Work out the finished part from the listing and answer in its coordinate system (mm). Face numbers are marked on the shaded views. A direction names the side the tool comes from. Round coordinates to 2 decimals unless told otherwise and drop trailing zeros. Loops run counter-clockwise (first coordinate to the right, second up) from the corner with the lowest first, then second, coordinate; pieces in that order, holes last. Notation, with made-up numbers: (-12.5, -27) -> (36.5, -27) arc R25 cw to (36.5, -11) -> close; hole circle Ø7 at (57.25, 84.25). An arc over 180 degrees is marked (long way). Use one line per item in the form item = value.
```python
from build123d import *

# Parameters (mm, degrees)
F0_R     = 6.5
F1_DEPTH = 25
F3_DEPTH = 40
F4_R     = 19.99999
F5_R     = 7
F6_DEPTH = 25


# Not quite as in the source:
# - a fillet or chamfer is up to 0.001 mm smaller than in the source, because OpenCascade refuses the exact size


with BuildPart() as f1:
    # F0 (on Front) → F1 (new body)
    with BuildSketch(Plane.XZ):
        with BuildLine():
            Line((0, -28.0120762104), (0, 51.4879237896))
            Line((0, 51.4879237896), (-45, 51.4879237896))
            Line((-45, 51.4879237896), (-55, 40.4879237896))
            Line((-55, 40.4879237896), (-55, 10.4879237896))
            Line((-55, 10.4879237896), (-22, -51.5120762104))
            Line((-22, -51.5120762104), (0, -51.5120762104))
            Line((0, -51.5120762104), (0, -41.0120762104))
            ThreePointArc((0, -41.0120762104), (-6.5, -34.5120762104), (0, -28.0120762104))
        make_face()
        with Locations((-38, 22.4879237896)):
            Circle(F0_R, mode=Mode.SUBTRACT)
        with BuildLine():
            Line((45, 51.4879237896), (0, 51.4879237896))
            Line((0, 51.4879237896), (0, -28.0120762104))
            ThreePointArc((0, -28.0120762104), (6.5, -34.5120762104), (0, -41.0120762104))
            Line((0, -41.0120762104), (0, -51.5120762104))
            Line((0, -51.5120762104), (22, -51.5120762104))
            Line((22, -51.5120762104), (55, 10.4879237896))
            Line((55, 10.4879237896), (55, 40.4879237896))
            Line((55, 40.4879237896), (45, 51.4879237896))
        make_face()
        with Locations((38, 22.4879237896)):
            Circle(F0_R, mode=Mode.SUBTRACT)
    extrude(amount=F1_DEPTH)

    # F2 (on face) → F3 (join)
    with BuildSketch(Plane(origin=(0, 0, 0), x_dir=(-1, 0, 0), z_dir=(0, 1, 0))):
        Polygon((7, 108.4879237896), (0, 108.4879237896), (-7, 108.4879237896), (-7, 47.4879237896), (-45, 47.4879237896), (-45, 39.4879237896), (-7, 39.4879237896), (-7, -14.5120762104), (0, -14.5120762104), (7, -14.5120762104), (7, 39.4879237896), (45, 39.4879237896), (45, 47.4879237896), (7, 47.4879237896), align=None)
    extrude(amount=F3_DEPTH)

    # F4 (radius 20 in the source; OpenCascade refuses exactly that, so slightly less here)
    f4_edges = [f1.edges().sort_by_distance(p)[0] for p in [
        (0, 0, 108.487924),
        (0, 40, 108.487924),
    ]]
    fillet(f4_edges, radius=F4_R)

    # F5 (on face) → F6 (cut)
    with BuildSketch(Plane.YZ.offset(7)):
        with Locations((20, 88.4879237896)):
            Circle(F5_R)
        Polygon((40, -14.5120762104), (40, 24.4879237896), (17, -14.5120762104), align=None)
    extrude(amount=-F6_DEPTH, mode=Mode.SUBTRACT)


solid = f1.part
```
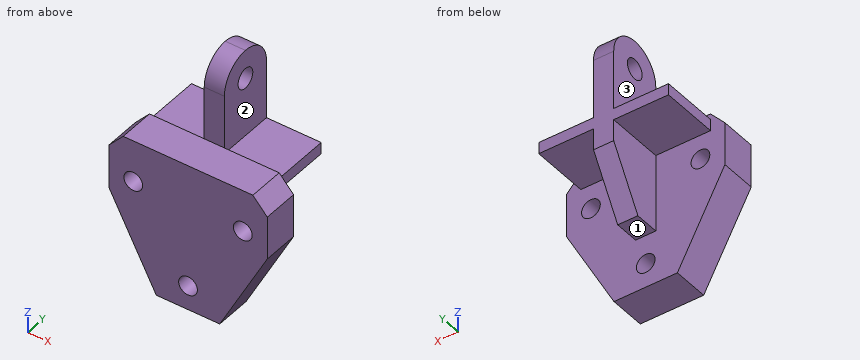
(1) Find section D-D, the plane z = 6. Write down the section's boundary in (x, y), then the cut area to 3 significant figures.
Completed:
outline = (-52.61, -25) -> (52.61, -25) -> (52.61, 0) -> (7, 0) -> (7, 29.1) -> (-7, 29.1) -> (-7, 0) -> (-52.61, 0) -> close
area = 3,040 mm2
(2) Find section C-C, the plane x = -38. Write down the section's boundary in (y, z).
Completed:
outline = (-25, -21.45) -> (0, -21.45) -> (0, 15.99) -> (-25, 15.99) -> close; (-25, 28.99) -> (0, 28.99) -> (0, 39.49) -> (40, 39.49) -> (40, 47.49) -> (0, 47.49) -> (0, 51.49) -> (-25, 51.49) -> close
(3) Consider L1, parallel to X at y = -10, z = 25; L2, parallel to Y at x = -29, z = -25.5; L3, parallel to Z at x = 25, y = 18.5. Determine where each line is inside the solid, lowest interval first.
Completed:
L1 = -55 to -43.99, -32.01 to 32.01, 43.99 to 55
L2 = -25 to 0
L3 = 39.49 to 47.49
(4) For the marked faces 1, 2 and 3, determine the directions among +Z, -Z, +X, -X, +Y, -Y from which every point of the face is accessible in a straight line to the end or side of a thin tool.
Completed:
face_1 = -Z, +X, -X, +Y
face_2 = +Z, +X, +Y
face_3 = +Z, -X, +Y
(5) Find section A-A, the plane x = 0. State how many separate pieces and enclosed holes the cut face has, then the cut area to 3 significant figures.
Completed:
separate_pieces = 2
enclosed_holes = 1
area = 6,400 mm2
(6) Find section B-B, the plane y = 22.5. Write down the section's boundary in (x, z), then the cut area to 3 significant figures.
Completed:
outline = (-45, 39.49) -> (-7, 39.49) -> (-7, -5.19) -> (7, -5.19) -> (7, 39.49) -> (45, 39.49) -> (45, 47.49) -> (7, 47.49) -> (7, 81.95) -> (-7, 81.95) -> (-7, 47.49) -> (-45, 47.49) -> close; (-7, 95.03) -> (7, 95.03) -> (7, 108.33) -> (-7, 108.33) -> close
area = 2,010 mm2
(7) Given P1, Ø3, axis at x = 27.5, y = 32.5, coming from the -Z side; P2, Ø12, axis at x = 0.5, z = -7.5, coming from the +Y side; P3, Ø12, axis at y = 26, z = 22, coming from the -X side; P4, Ø21, axis at x = 0, z = -34.51, coming from the -Y side, each flat-ended and moving along its own axis, determine where each tip first touches the part or whether it passes through.
Completed:
P1 = 39.49
P2 = 24.67
P3 = -7
P4 = -25
